Read the model definition and answer for the solid it produces. Units are mm, in the model's axes. Face numbers are marked on the shaded views. A direction names the side the tool comes from. Round coordinates to 2 decimals unless told otherwise and drop trailing zeros. Write each loop counter-clockwise with the first axis right and the second up, starting at its lowest first coordinate (ties: lowest second). Pieces come first, ordered by that corner, then holes.
from build123d import *

# Parameters (mm, degrees)
F1_DEPTH = 25.4
F2_R     = 90.4875
F3_DEPTH = 2.38125
F4_R     = 4.7625
F5_DEPTH = 12.7


with BuildPart() as f1:
    # F0 (on Front) → F1 (new body, symmetric)
    with BuildSketch(Plane.XZ):
        with BuildLine():
            Line((0, -9.525), (0, -44.45))
            Line((0, -44.45), (38.1, -44.45))
            ThreePointArc((38.1, -44.45), (56.251929, 0), (38.1, 44.45))
            Line((38.1, 44.45), (0, 44.45))
            Line((0, 44.45), (0, 9.525))
            ThreePointArc((0, 9.525), (9.525, 0), (0, -9.525))
        make_face()
    extrude(amount=F1_DEPTH, both=True)

    # F2 (on Front) → F3 (cut, symmetric)
    with BuildSketch(Plane.XZ):
        with Locations((107.95, 0)):
            Circle(F2_R)
    extrude(amount=F3_DEPTH, both=True, mode=Mode.SUBTRACT)

    # F4 (on Right) → F5 (join)
    with BuildSketch(Plane.YZ):
        with Locations((12.7, 31.75)):
            Circle(F4_R)
        with Locations((-12.7, 31.75)):
            Circle(F4_R)
        with Locations((-12.7, -31.75)):
            Circle(F4_R)
        with Locations((12.7, -31.75)):
            Circle(F4_R)
    extrude(amount=-F5_DEPTH)


solid = f1.part
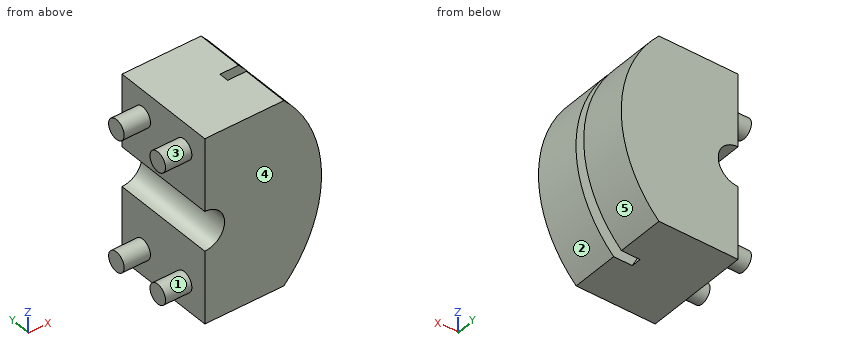
Q1. Section A-A (x = 31) is taken. Determine the outline of the cut face in (y, z).
Verdict:
outline: (-25.4, -44.45) - (-2.38, -44.45) - (-2.38, 44.45) - (-25.4, 44.45) - close; (2.38, -44.45) - (25.4, -44.45) - (25.4, 44.45) - (2.38, 44.45) - close
Q2. Determine the mould class of the marked faces 3, 4 and 5 for opening direction Z: pulls with the +Z half, pulls with the -Z half, needs draft (parallel to the pull), parting line crosses it, or undercut.
Verdict:
face 3: undercut
face 4: needs draft
face 5: parting line crosses it
Q3. Section D-D (x = 49.5) is taken. Determine the outline of the cut face in (y, z), then the cut area to 3 significant figures.
Verdict:
outline: (-25.4, -28.49) - (-2.38, -28.49) - (-2.38, 28.49) - (-25.4, 28.49) - close; (2.38, -28.49) - (25.4, -28.49) - (25.4, 28.49) - (2.38, 28.49) - close
area: 2,620 mm2
Q4. Flat-ended cylindrical pins translate along their axes: pin 1 Ø1 at (y, z) = (-16.5, 8) entering from -X; pin 2 Ø2 at (x, y) = (-2, -9) entering from +Z; pin 3 Ø8 at (y, z) = (-11.5, 2.5) entering from -X. Find the tip coordinate at first contact, or state that the pin passes through.
Verdict:
pin 1: stops at x = 4.3
pin 2: stops at z = 35.67
pin 3: stops at x = 6.96
Q5. Section B-B (z = 0) is taken. Determine the outline of the cut face in (x, y) (1 decimal), then the cut area to 3 significant figures.
Verdict:
outline: (9.5, -25.4) - (56.3, -25.4) - (56.3, -2.4) - (17.5, -2.4) - (17.5, 2.4) - (56.3, 2.4) - (56.3, 25.4) - (9.5, 25.4) - close
area: 2,190 mm2
Q6. Which of the six approach directions +Z, -Z, +X, -X, +Y, -Y give full straight-line access (tool end or side, diameter ignored) to the marked faces 1 and 2?
Verdict:
face 1: -X
face 2: +X, +Y, -Y
Q7. Straight lines are drawn through the part: probe 1 along Y at (x, z) = (32.5, -11.5); probe 2 along Y at (x, z) = (-1, 28); probe 3 along Z at (x, y) = (26, 2). For each, find the intervals that lie inside material, in ascending order.
Verdict:
probe 1: y = -25.4 to -2.38, 2.38 to 25.4
probe 2: y = -15.64 to -9.76, 9.76 to 15.64
probe 3: z = -44.45 to -38.37, 38.37 to 44.45
